Geometry: final body of the model. Coordinates: model frame, mm. Face numbers are marked on the shaded views. A direction names the side the tool comes from. Give positions to 0.01 mm unless a question says otherwise; leave off trailing zeros. Write each loop counter-clockwise with the first axis right and the second up, starting at its lowest first coordinate (ties: lowest second). Pieces come first, ordered by that corner, then holes. Notation, with made-up numbers: (85, 88.5) -> (120, 88.5) arc R15 cw to (120, 104.5) -> close; hole circle Ø4 at (87.25, 46). An arc over 180 degrees is marked (long way). Answer as a JSON object with one key per item and string values. Group by question number.
(1) Set-up query: the marked faces 1 and 2. Return all of +Z, -Z, +X, -X, +Y, -Y with unobstructed straight access to the full face (end or side cutting, diameter ignored); none if empty.
(2) Section query A-A on y = 0. Output: boundary loops of the cut face in (x, z) (3 decimals).
(3) Contact query for flat-ended pins moving along their axis: pin 1 Ø8 at (y, z) = (9.5, -17) entering from +X; pin 2 Ø10 at (y, z) = (6.5, -23) entering from -X; pin 3 Ø6 at (x, y) = (-0.5, 11.5) entering from -Z; pin 4 Ø15 at (x, y) = (-6.5, -5) entering from -Z. Output: stop coordinate, or through.
(4) Section query D-D on z = -25.5. Output: boundary loops of the cut face in (x, y).
(5) Section query C-C on z = -7. Output: boundary loops of the cut face in (x, y), plus the area to 3 significant figures.
(6) Material intervals for probe 1 along Z at (x, y) = (8.5, 11) (3 decimals); probe 2 along X at (y, z) = (0.5, -7.5), sorted ascending.
from build123d import *

# Parameters (mm, degrees)
SKETCH1_R           = 15.24
BOSS_EXTRUDE1_DEPTH = 0.635
SKETCH2_R           = 1.7272
BOSS_EXTRUDE2_DEPTH = 22.86
SKETCH3_R           = 0.6096
BOSS_EXTRUDE3_DEPTH = 8.89


with BuildPart() as part:
    # Sketch1 → Boss-Extrude1 (new body)
    with BuildSketch(Plane.XY):
        Circle(SKETCH1_R)
    extrude(amount=BOSS_EXTRUDE1_DEPTH)

    # Sketch2 → Boss-Extrude2 (add)
    with BuildSketch(Plane(origin=(0, 0, 0), x_dir=(-1, 0, 0), z_dir=(0, 0, -1))):
        Circle(SKETCH2_R)
    extrude(amount=BOSS_EXTRUDE2_DEPTH)

    # Sketch3 → Boss-Extrude3 (add)
    with BuildSketch(Plane(origin=(0, 0, -22.86), x_dir=(-1, 0, 0), z_dir=(0, 0, -1))):
        Circle(SKETCH3_R)
    extrude(amount=BOSS_EXTRUDE3_DEPTH)


solid = part.part
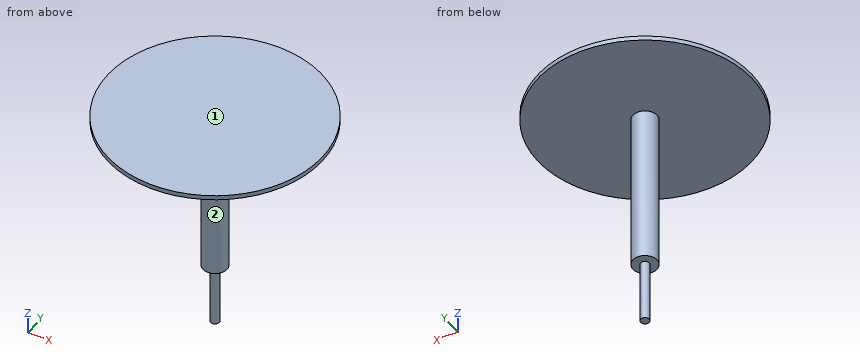
Answer list:
{
 "1": {"face 1": "+Z, +X, -X, +Y, -Y", "face 2": "-Z"},
 "2": {"outline": "(-15.24, 0) -> (-1.727, 0) -> (-1.727, -22.86) -> (-0.61, -22.86) -> (-0.61, -31.75) -> (0.61, -31.75) -> (0.61, -22.86) -> (1.727, -22.86) -> (1.727, 0) -> (15.24, 0) -> (15.24, 0.635) -> (-15.24, 0.635) -> close"},
 "3": {"pin 1": "through", "pin 2": "x = -0.85", "pin 3": "z = 0", "pin 4": "z = -22.86"},
 "4": {"outline": "circle Ø1.22 at (0, 0)"},
 "5": {"outline": "circle Ø3.45 at (0, 0)", "area": "9.37 mm2"},
 "6": {"probe 1": "0 to 0.635", "probe 2": "-1.65 to 1.65"}
}
